Study the drawing (mm; zero at the part's minimum x, y, z) and answer. A direction names the side the tool comes from. Give positions to 0.01 mm unless a question says otherwise; leave off trailing zeros. Loops run counter-clockwise (first coordinate to the right, second up) from the corner with the lowest first, then second, coordinate; pieces in that order, holes last. Notation, with made-up numbers: (-36, 85) - (-16, 85) arc R5 cw to (-16, 90) - close; hole circle Ø2 at (-29.75, -35.75). An arc over 180 degrees is marked (long way). Write item = value, one per line. Start each with the question number.
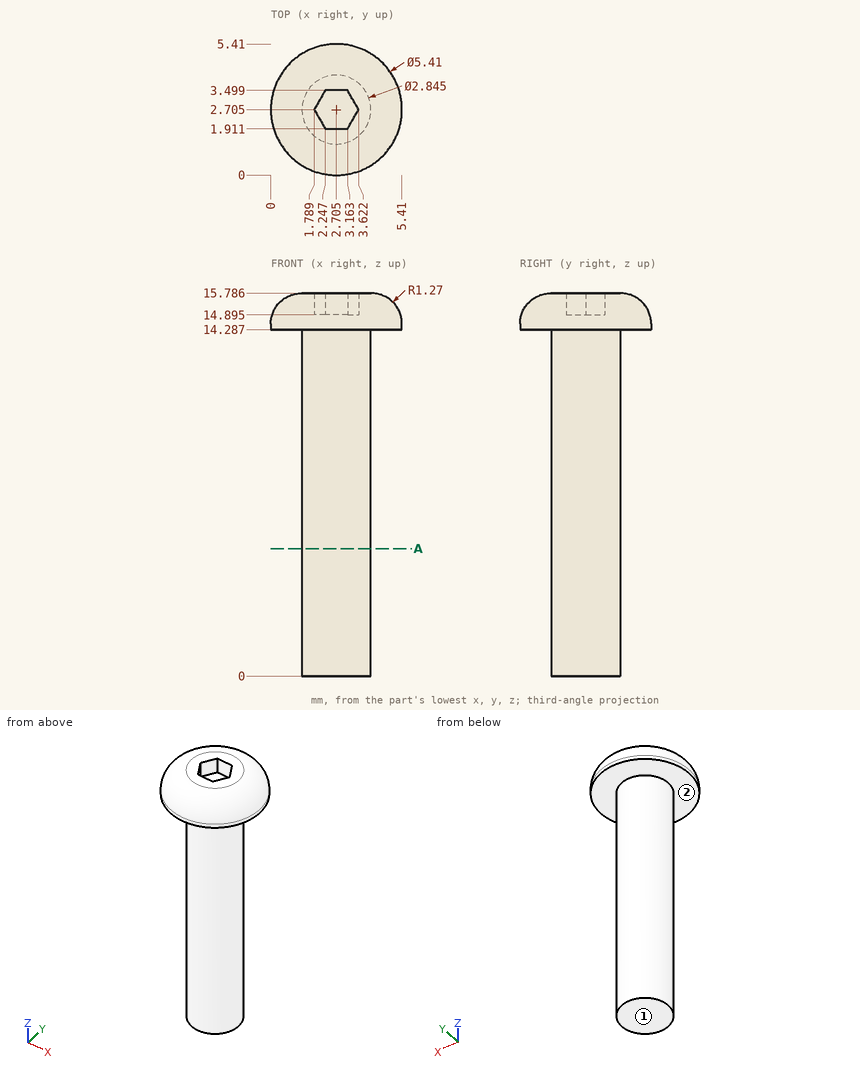
1. A cutting plane is placed at A-A on z = 5.25. Give the vertices of the cut face in (x, y) (1 decimal).
2. Consider line 1 along Z through (x, y) = (2.45, 2.05) (1 decimal); line 2 along Y through (x, z) = (2.45, 1.75) (1 decimal); line 3 along Z through (x, y) = (4.55, 3). Determine where each line is inside the solid, lowest interval first. Write a range as [from, to].
3. Given P1, Ø3, axis at y = 2, z = 2, coming from the -X side; P2, Ø2, axis at x = 4, y = 0.5, coming from the +Z side; P3, Ø1.5, axis at y = 4.5, z = 4, coming from the -X side, each flat-ended and moving along its own axis, determine where each tip first touches the part or whether it passes through.
4. A tool of negligible diameter and unlimited length cuts with its end or side. For the marked faces 1 and 2, from which of +Z, -Z, +X, -X, +Y, -Y can it reach the whole face along a straight path? Write none if from no direction.
Reply:
q1.outline = circle Ø2.8 at (2.7, 2.7)
q2.line_1 = [0, 14.9]
q2.line_2 = [1.3, 4.1]
q2.line_3 = [14.29, 15.71]
q3.P1 = 1.28
q3.P2 = 15.78
q3.P3 = 1.74
q4.face_1 = -Z, +X, -X, +Y, -Y
q4.face_2 = -Z
